Here's how the part is built. I have some questions about the finished solid (model axes, mm). Face numbers are marked on the shaded views. A direction names the side the tool comes from. Round coordinates to 2 decimals unless told otherwise and drop trailing zeros. Write each loop counter-clockwise with the first axis right and the second up, starting at its lowest first coordinate (ties: lowest second). Pieces come first, ordered by that corner, then holes. Notation, with made-up numbers: M 65,3.25 L 70,3.25 A5 ccw 70,12.25 Z; hole C 39,-2.75 d10. An arc over 180 degrees is marked long. Use a Markdown table: item, result. Add a question column.
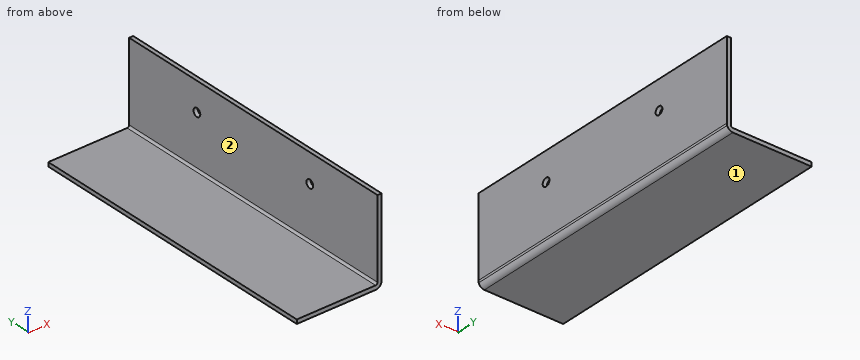
```python
from build123d import *

# Parameters (mm, degrees)
SKETCH2_W              = 60
SKETCH2_H              = 110
BASE_FLANGE1_DEPTH     = 1.5
SKETCHED_BEND1_DEPTH   = 110
SKETCHED_BEND1_2_DEPTH = 110
F_3_0MM_DOWEL_HOLE2_D  = 3


# Read off the part's stored shape, not the designer's step: Sketched Bend1
# Sheet-metal steps are written as plain solids
with BuildPart() as part:
    # Sketch2 → Base-Flange1 (new body)
    with BuildSketch(Plane.XY):
        with Locations((30, 55)):
            Rectangle(SKETCH2_W, SKETCH2_H)
    extrude(amount=-BASE_FLANGE1_DEPTH)

    # Sketched Bend1 outline → Sketched Bend1 (cut)
    with BuildSketch(Plane(origin=(0, 0, 0), x_dir=(1, 0, 0), z_dir=(0, 1, 0))):
        with BuildLine():
            ThreePointArc((28.83242709, 1.5), (30.127591172, 1.086838938), (30.944250946, 0))
            Line((30.944250946, 0), (60, 0))
            Line((60, 0), (60, 1.5))
            Line((60, 1.5), (28.83242709, 1.5))
        make_face()
    extrude(amount=SKETCHED_BEND1_DEPTH, mode=Mode.SUBTRACT)

    # Sketched Bend1 2 outline → Sketched Bend1 2 (add)
    with BuildSketch(Plane(origin=(0, 0, 0), x_dir=(1, 0, 0), z_dir=(0, 1, 0))):
        with BuildLine():
            Line((29.56902709, -0.7366), (29.56902709, -29.56902709))
            Line((29.56902709, -29.56902709), (31.06902709, -29.56902709))
            Line((31.06902709, -29.56902709), (31.06902709, -0.7366))
            ThreePointArc((31.06902709, -0.7366), (31.037612433, -0.363053267), (30.944250946, 0))
            Line((30.944250946, 0), (28.83242709, 0))
            ThreePointArc((28.83242709, 0), (29.353281945, -0.215745145), (29.56902709, -0.7366))
        make_face()
    extrude(amount=SKETCHED_BEND1_2_DEPTH)

    # Ø3.0mm Dowel Hole2 (through all)
    with Locations(Plane(origin=(29.56902709, -1.119987894, 38.304969563), x_dir=(0, 0, 1), z_dir=(-1, 0, 0))):
        with Locations((-19.237938753, 81.119987894), (-19.237938753, 31.119987894)):
            Hole(F_3_0MM_DOWEL_HOLE2_D / 2)


solid = part.part
```
Item 1: For pin 1 Ø3 at (x, y) = (4, 22) entering from +Z; pin 2 Ø6 at (x, z) = (6.5, 3.5) entering from +Y; pin 3 Ø4 at (y, z) = (47, 16) entering from -X, each with a flat end and sliding along its axis, tell me the tip position at first contact or that it passes through.
Item 2: Imagine slicing it at C-C on x = 9. List the corners of the cut face in (y, z) for me.
Item 3: On a 3-axis mill with a long thin cutter (end or side, diameter ignored), from which of +Z, -Z, +X, -X, +Y, -Y can I reach the whole of each face in a straight line? I mean the marked faces 1 and 2. Say none if no direction works.
Item 4: Imagine slicing it at B-B on y = 50.5. List the corners of the cut face in (x, z) for me, plus the area to 3 significant figures.
Item 5: Imagine slicing it at D-D on z = 11.5. List the corners of the cut face in (x, y) for me.
Item 6: I need wall thicknesses on probe 1 along X at (y, z) = (48.5, 7); probe 2 along Z at (x, y) = (22, 9); probe 3 along Z at (x, y) = (30.5, 80). Which ranges of each line are inside material? Lowest first, please. Write a range as from..to.
Item 7: Imagine slicing it at A-A on y = 30. List the corners of the cut face in (x, z) for me, plus the area to 3 significant figures.
The answers:
| question | item | result |
|---|---|---|
| 1 | pin 1 | z = 0 |
| 1 | pin 2 | through |
| 1 | pin 3 | x = 29.57 |
| 2 | outline | M 0,-1.5 L 110,-1.5 L 110,0 L 0,0 Z |
| 3 | face 1 | -Z, +X, -X, +Y, -Y |
| 3 | face 2 | +Z, -X, +Y, -Y |
| 4 | outline | M 0,-1.5 L 28.83,-1.5 A2.24 ccw 31.07,0.74 L 31.07,29.57 L 29.57,29.57 L 29.57,0.74 A0.74 cw 28.83,0 L 0,0 Z |
| 4 | area | 90.0 mm² |
| 5 | outline | M 29.57,0 L 31.07,0 L 31.07,110 L 29.57,110 Z |
| 6 | probe 1 | 29.57..31.07 |
| 6 | probe 2 | -1.5..0 |
| 6 | probe 3 | -0.75..17.57, 20.57..29.57 |
| 7 | outline | M 0,-1.5 L 28.83,-1.5 A2.24 ccw 31.07,0.74 L 31.07,17.57 L 29.57,17.57 L 29.57,0.74 A0.74 cw 28.83,0 L 0,0 Z; M 29.57,20.57 L 31.07,20.57 L 31.07,29.57 L 29.57,29.57 Z |
| 7 | area | 85.5 mm² |
